Part model, mm, in its own coordinate system. Face numbers are marked on the shaded views. A direction names the side the tool comes from. Give positions to 0.01 mm unless a question says otherwise; leave off trailing zeros. Loops run counter-clockwise (first coordinate to the right, second up) from the corner with the lowest first, then second, coordinate; pieces in that order, holes last. Notation, with made-up numbers: (66, -34) -> (122, -34) arc R23 cw to (122, -7) -> close; hole circle Ø9 at (-6, 55). An arc over 180 degrees is marked (long way). One line per question, with ' | ' between items.
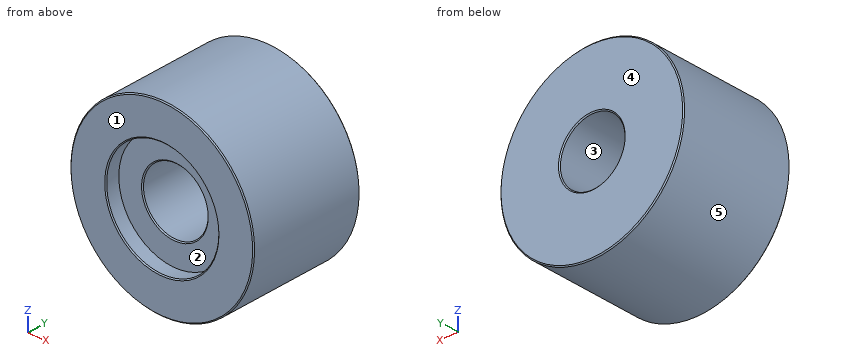
```python
from build123d import *

# Parameters (mm, degrees)
MAIN_DIMENSIONS_SKETCH_R   = 9
MAIN_DIMENSIONS_SKETCH_R_2 = 5.5
MAIN_DIMENSIONS_SKETCH_R_3 = 3.16865
BODY_DEPTH                 = 10
SKETCH1_3_R                = 9
SKETCH1_3_R_2              = 5.5
LIP_DEPTH                  = 1.4
BREAK_EDGES_SIZE           = 0.1


with BuildPart() as part:
    # main_dimensions_sketch → body (new body)
    with BuildSketch(Plane(origin=(0, 0, 0), x_dir=(1, 0, 0), z_dir=(0, 1, 0))):
        Circle(MAIN_DIMENSIONS_SKETCH_R)
        Circle(MAIN_DIMENSIONS_SKETCH_R_2, mode=Mode.SUBTRACT)
        Circle(MAIN_DIMENSIONS_SKETCH_R_2)
        Circle(MAIN_DIMENSIONS_SKETCH_R_3, mode=Mode.SUBTRACT)
    extrude(amount=BODY_DEPTH)

    # Sketch1_3 → lip (add)
    with BuildSketch(Plane(origin=(0, 0, 0), x_dir=(1, 0, 0), z_dir=(0, 1, 0))):
        Circle(SKETCH1_3_R)
        Circle(SKETCH1_3_R_2, mode=Mode.SUBTRACT)
    extrude(amount=-LIP_DEPTH)

    # break_edges
    break_edges_edges = [part.edges().sort_by_distance(p)[0] for p in [
        (-3.16865, 0, 0),
        (-9, 10, 0),
        (-3.16865, 10, 0),
        (-9, -1.4, 0),
        (-5.5, -1.4, 0),
    ]]
    chamfer(break_edges_edges, length=BREAK_EDGES_SIZE)


solid = part.part
```
1) Tool access for the marked faces 1 and 2: list every direction of +Z, -Z, +X, -X, +Y, -Y with a clear straight run to the whole face (end or side of a thin tool).
Found:
face 1: +Z, -Z, +X, -X, -Y | face 2: -Y
2) Drill centre lines: line 1 (X direction, y = -0.25, z = 0); line 2 (X direction, y = 3.75, z = 2.5). Where is each one in solid material? Low to high.
Found:
line 1: -9 to -5.5, 5.5 to 9 | line 2: -8.65 to -1.95, 1.95 to 8.65
3) Pull direction X, two halves, no side cores. Call the marked faces 3, 4 and 5: pulls with the +X half, pulls with the -X half, needs draft (parallel to the pull), parting line crosses it, or undercut.
Found:
face 3: undercut | face 4: needs draft | face 5: parting line crosses it
4) Pin check, flat tips, straight feed: P1, Ø3, axis at x = -6.5, y = 5, coming from the -Z side; P2, Ø10, axis at x = 0, z = 0, coming from the -Y side; P3, Ø4, axis at x = -2.5, y = 3.5, coming from the -Z side; P4, Ø5, axis at x = 0, z = 0, coming from the -Y side. Stop position of each tip, or through.
Found:
P1: z = -7.48 | P2: y = 0 | P3: z = -8.99 | P4: through
5) Saw through at B-B (x = 0). Give the cut face in (y, z).
Found:
outline: (-1.4, -8.9) -> (-1.3, -9) -> (9.9, -9) -> (10, -8.9) -> (10, -3.27) -> (9.9, -3.17) -> (0.1, -3.17) -> (0, -3.27) -> (0, -5.5) -> (-1.3, -5.5) -> (-1.4, -5.6) -> close; (-1.4, 5.6) -> (-1.3, 5.5) -> (0, 5.5) -> (0, 3.27) -> (0.1, 3.17) -> (9.9, 3.17) -> (10, 3.27) -> (10, 8.9) -> (9.9, 9) -> (-1.3, 9) -> (-1.4, 8.9) -> close
6) Saw through at C-C (y = 3). Give the cut face in (x, z).
Found:
outline: circle Ø18 at (0, 0); hole circle Ø6.34 at (0, 0)
7) Saw through at A-A (z = 0). Give the cut face in (x, y).
Found:
outline: (-9, -1.3) -> (-8.9, -1.4) -> (-5.6, -1.4) -> (-5.5, -1.3) -> (-5.5, 0) -> (-3.27, 0) -> (-3.17, 0.1) -> (-3.17, 9.9) -> (-3.27, 10) -> (-8.9, 10) -> (-9, 9.9) -> close; (3.17, 0.1) -> (3.27, 0) -> (5.5, 0) -> (5.5, -1.3) -> (5.6, -1.4) -> (8.9, -1.4) -> (9, -1.3) -> (9, 9.9) -> (8.9, 10) -> (3.27, 10) -> (3.17, 9.9) -> close
